Check sheet for the modelled part. Datum: model origin and axes. Units: mm. A direction names the side the tool comes from. Give positions to 0.01 mm unless a question says otherwise; leave off trailing zeros. Order: outer loops, then holes, each group sorted by start corner. A loop starts at its lowest first (then second) coordinate and runs counter-clockwise, first axis right, second up. Notation, with made-up numbers: (20.5, 38.5) -> (34.5, 38.5) arc R23 ccw to (34.5, 62.5) -> close; hole circle Ø10 at (-37.75, 29). An arc over 180 degrees is marked (long way). One line per question, with ' | ' between items. Start each with the question number.
from build123d import *

# Parameters (mm, degrees)
SKETCH1_R           = 15
SKETCH1_R_2         = 13.5
BOSS_EXTRUDE1_DEPTH = 0.75
CIRPATTERN1_COUNT   = 6


with BuildPart() as part:
    # Sketch1 → Boss-Extrude1 (new, symmetric)
    with BuildSketch(Plane.XY):
        Circle(SKETCH1_R)
        Circle(SKETCH1_R_2, mode=Mode.SUBTRACT)
    boss_extrude1 = extrude(amount=BOSS_EXTRUDE1_DEPTH, both=True)

    # CirPattern1: Boss-Extrude1 ×6 about axis
    cirpattern1_axis = Axis((0, 0, 0), (1, 0, 0))
    for i in range(1, CIRPATTERN1_COUNT):
        add(boss_extrude1.rotate(cirpattern1_axis, i * 360 / CIRPATTERN1_COUNT))


solid = part.part
1. Cross-section at C-C on y = -5.75. Give the number of separate pieces and of enclosed holes in the cut face, and give its area (3 significant figures).
2. Mould release check, pull along Z, two halves, no side actions. Record for faces 3 (the face through (0.297, 13.497, -0.01)), 4 (the face through (0.32, 7.49, 12.99)): +Z half, -Z half, draft (parallel to the pull), parting line (faces both ways), or undercut.
3. Scan lines: probe 1 along Z at (x, y) = (11, -9); probe 2 along X at (y, z) = (-10.25, 0); probe 3 along X at (y, z) = (8.75, -0.5). Record each from-to range of solid material in increasing order.
4. Tool access check on faces 1 (the face through (0, -15, 0)), 2 (the face through (0.297, -6.739, 11.694)). Record the directions out of +Z, -Z, +X, -X, +Y, -Y that give a thin tool (end or side, any length) a straight path to the whole face; none if there is none.
5. Cross-section at A-A on y = 9. Record the boundary of the cut face in (x, z), and give its area (3 significant figures).
6. Go/stop test with flat-tipped pins: pin 1 (5 mm diameter, centred on x = 8, z = -7, fed in from -Y); pin 2 (7 mm diameter, centred on x = 0, y = 10.5, fed in from -Z); pin 3 (12 mm diameter, centred on x = 10, y = 11.5, fed in from +Z). Record where each tip stops, or that it passes through.
7. Cross-section at B-B on x = 11.5. Record the boundary of the cut face in (y, z), and give its area (3 significant figures).
Response values:
1) separate pieces: 6 | enclosed holes: 0 | area: 36.7 mm²
2) face 3: undercut | face 4: +Z half
3) probe 1: z = -0.75 to 0.75 | probe 2: x = -10.95 to -8.79, 8.79 to 10.95 | probe 3: x = -12.18 to -10.28, 10.28 to 12.18
4) face 1: +Z, -Z, -Y | face 2: none
5) outline: (-12, -0.75) -> (-10.06, -0.75) -> (-10.06, 0.75) -> (-12, 0.75) -> close; (10.06, -0.75) -> (12, -0.75) -> (12, 0.75) -> (10.06, 0.75) -> close | area: 5.81 mm²
6) pin 1: stops at y = -6.35 | pin 2: stops at z = -13.28 | pin 3: stops at z = 11.82
7) outline: (-9.63, -0.75) -> (-7.07, -0.75) -> (-7.07, 0.75) -> (-9.63, 0.75) -> close; (-5.46, -7.97) -> (-4.17, -8.72) -> (-2.89, -6.5) -> (-4.19, -5.75) -> close; (-5.46, 7.97) -> (-4.19, 5.75) -> (-2.89, 6.5) -> (-4.17, 8.72) -> close; (2.89, -6.5) -> (4.17, -8.72) -> (5.46, -7.97) -> (4.19, -5.75) -> close; (2.89, 6.5) -> (4.19, 5.75) -> (5.46, 7.97) -> (4.17, 8.72) -> close; (7.07, -0.75) -> (9.63, -0.75) -> (9.63, 0.75) -> (7.07, 0.75) -> close | area: 23.0 mm²
